Check sheet for the drawn part. Datum: minimum x, y, z corner. Units: mm. A direction names the side the tool comes from. Coordinates: 2 decimals unless noted, no trailing zeros. Order: outer loops, then holes, each group sorted by start corner. A loop starts at its lowest first (then second) coordinate and runs counter-clockwise, first axis right, second up.
1. Thickness scan on line 1 (X direction, y = 8.5, z = 2); line 2 (Z direction, x = 66, y = 2); line 3 (X direction, y = 2.75, z = 20). Record the ranges inside material, lowest first.
2. Cross-section at B-B (x = 43). Enter the section's corners in (y, z).
3. Cross-section at C-C (y = 3.25). Enter the section's corners in (x, z).
4. Gauge pin test, flat end, axial feed: pin 1 Ø4 at (y, z) = (9, 23.5) entering from -X. Record the tip position at first contact, or that the pin passes through.
5. Cross-section at D-D (z = 12). Enter the section's corners in (x, y), then the cut area to 3 significant figures.
6. Draft check along Z on the marked faces 6, 7 and 8. Enter one of: released by +Z, released by -Z, zero draft, split by the parting line, or undercut.
7. Cross-section at A-A (z = 24). Enter the section's corners in (x, y).
8. Set-up check for the marked faces 1, 2, 3, 4 and 5: record each of +Z, -Z, +X, -X, +Y, -Y from which the full face is reachable in a straight line by a thin tool's end or side.
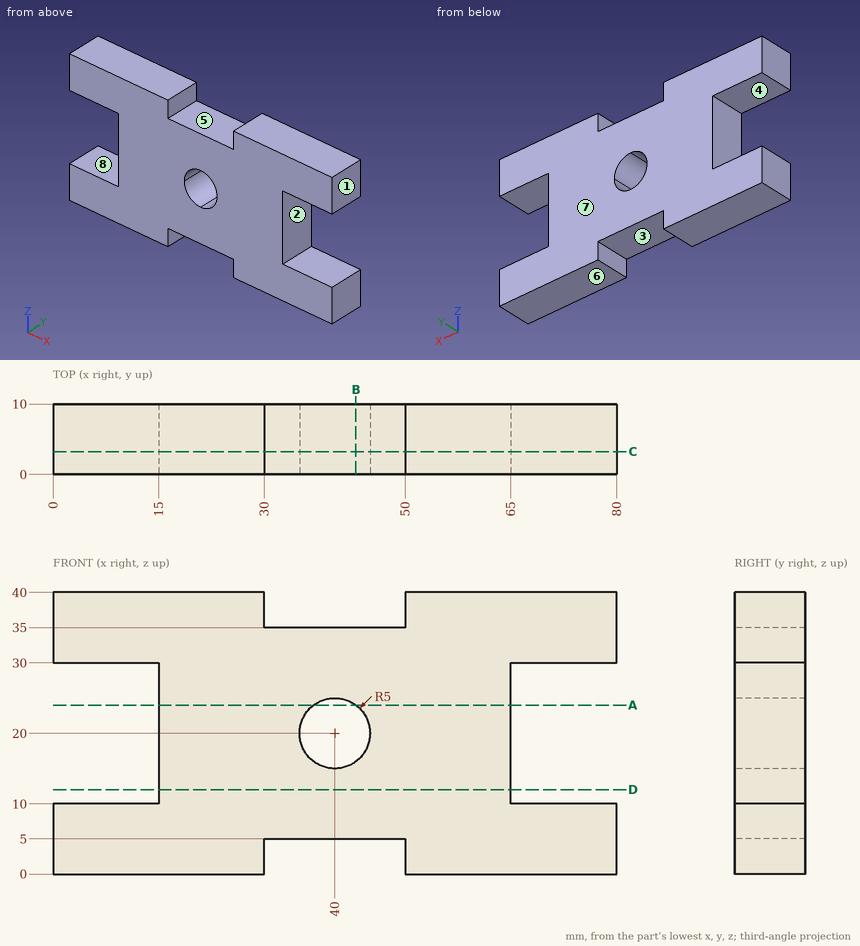
Data:
1. line 1: x = 0 to 30, 50 to 80
1. line 2: z = 0 to 10, 30 to 40
1. line 3: x = 15 to 35, 45 to 65
2. outline: (0, 5) - (10, 5) - (10, 16) - (0, 16) - close; (0, 24) - (10, 24) - (10, 35) - (0, 35) - close
3. outline: (0, 0) - (30, 0) - (30, 5) - (50, 5) - (50, 0) - (80, 0) - (80, 10) - (65, 10) - (65, 30) - (80, 30) - (80, 40) - (50, 40) - (50, 35) - (30, 35) - (30, 40) - (0, 40) - (0, 30) - (15, 30) - (15, 10) - (0, 10) - close; hole circle Ø10 at (40, 20)
4. pin 1: stops at x = 15
5. outline: (15, 0) - (65, 0) - (65, 10) - (15, 10) - close
5. area: 500 mm2
6. face 6: released by -Z
6. face 7: zero draft
6. face 8: undercut
7. outline: (15, 0) - (37, 0) - (37, 10) - (15, 10) - close; (43, 0) - (65, 0) - (65, 10) - (43, 10) - close
8. face 1: +Z, -Z, +X, +Y, -Y
8. face 2: +X, +Y, -Y
8. face 3: -Z, +Y, -Y
8. face 4: -X, +Y, -Y
8. face 5: +Z, +Y, -Y
